from build123d import *

# Parameters (mm, degrees)
SKETCH_1_R                      = 1.440775231
EXTRUDE_1_DEPTH                 = 5
SKETCH_3_W                      = 35
SKETCH_3_H                      = 4
EXTRUDE_2_DEPTH                 = 50
FILLET_1_R                      = 10
FILLET_2_R                      = 5
CUT_EXTRUDE_2_DEPTH             = 63.339794674
CUT_EXTRUDE_2_DEPTH_BACK        = 63.339794674
CUT_EXTRUDE_3_REACH             = 64.34
SKETCH_5_R                      = 1.7
SKETCH_5_W                      = 10
SKETCH_5_H                      = 2.5
CUT_EXTRUDE_3_DIRECTION_2_DEPTH = 63.339794674
FILLET_3_R                      = 0.5
FILLET_4_R                      = 1


with BuildPart() as part:
    # 草图1 → 凸台-拉伸1 (new body)
    with BuildSketch(Plane.XY):
        with BuildLine():
            Line((-26, -2.5), (26, -2.5))
            ThreePointArc((26, -2.5), (28.5, 0), (26, 2.5))
            Line((26, 2.5), (20, 5))
            Line((20, 5), (-20, 5))
            Line((-20, 5), (-26, 2.5))
            ThreePointArc((-26, 2.5), (-28.5, 0), (-26, -2.5))
        make_face()
        with Locations((-26, 0)):
            Circle(SKETCH_1_R, mode=Mode.SUBTRACT)
        with Locations(Location((26, 0, 0), (0, 0, 180))):
            Circle(SKETCH_1_R, mode=Mode.SUBTRACT)
    extrude(amount=EXTRUDE_1_DEPTH)

    # 草图3 → 凸台-拉伸2 (add)
    with BuildSketch(Plane.XY.offset(5)):
        Rectangle(SKETCH_3_W, SKETCH_3_H)
    extrude(amount=EXTRUDE_2_DEPTH)

    # 圆角1
    # the kernel refuses this fillet: 10 mm, written as the material it adds along each edge
    with BuildSketch(Plane(origin=(17.5, -2, 5), x_dir=(0, -1.0, 2.1849189124477904e-12), z_dir=(-1, 0, 0))) as fillet_1_piece_1:
        with BuildLine():
            CenterArc((10, 3.122498999), FILLET_1_R, 180, 18.194872339)
            Line((0, 3.122498999), (-0.2, 3.122498999))
            Line((-0.2, 3.122498999), (-0.2, 0))
            Line((-0.2, 0), (0, -0.2))
            ThreePointArc((0, -0.2), (0.25, -0.2), (0.31, -0.06244998))
            Line((0.31, -0.06244998), (0.5, 0))
        make_face()
    extrude(amount=35)

    # 圆角2
    # the kernel refuses this fillet: 5 mm, written as the material it adds along each edge
    with BuildSketch(Plane(origin=(-17.5, 2, 5), x_dir=(0, 0, 1), z_dir=(1, 0, 0))) as fillet_2_piece_1:
        with BuildLine():
            CenterArc((4.582575695, -5), FILLET_2_R, 90, 66.421821522)
            Line((0, -3), (-0.091651514, -2.96))
            ThreePointArc((-0.091651514, -2.96), (-0.1, -1.5), (-0.1, 0))
            Line((-0.1, 0), (0, 0.1))
            Line((0, 0.1), (4.582575695, 0.1))
            Line((4.582575695, 0.1), (4.582575695, 0))
        make_face()
    extrude(amount=35)

    # 草图4 → 切除-拉伸2 (cut, two sides: drawn at the far end of the back side and taken through both)
    with BuildSketch(Plane.XZ.offset(2).offset(-CUT_EXTRUDE_2_DEPTH_BACK)):
        Polygon((-17.5, 51), (-13.5, 55), (-17.5, 55), align=None)
        Polygon((-13.5, 23), (-17.5, 27), (-17.5, 5), (-15.5, 5.511275368), (-10.5, 5.511275368), (-7.888776369, 8.122498999), (-7.888776369, 20.122498999), (-10.5, 23), align=None)
        Polygon((17.5, 5), (17.5, 27), (13.5, 23), (10.5, 23), (7.888776369, 20.122498999), (7.888776369, 8.122498999), (10.5, 5.511275368), (15.5, 5.511275368), align=None)
        Polygon((17.5, 51), (17.5, 55), (13.5, 55), align=None)
    extrude(amount=CUT_EXTRUDE_2_DEPTH + CUT_EXTRUDE_2_DEPTH_BACK, mode=Mode.SUBTRACT)

    # 草图5 → 切除-拉伸3 (cut, up to next)
    with BuildSketch(Plane.XZ.offset(2), mode=Mode.PRIVATE) as cut_extrude_3_sk1:
        with Locations(Location((-11.5, 26.128065597, 0), (0, 0, 180))):
            Circle(SKETCH_5_R)
    cut_extrude_3_tool1 = extrude(cut_extrude_3_sk1.sketch, amount=-CUT_EXTRUDE_3_REACH, mode=Mode.PRIVATE) & part.part
    # 草图5 → 切除-拉伸3 (cut, up to next)
    with BuildSketch(Plane.XZ.offset(2), mode=Mode.PRIVATE) as cut_extrude_3_sk2:
        with Locations(Location((11.5, 26.128065597, 0), (0, 0, 180))):
            Circle(SKETCH_5_R)
    cut_extrude_3_tool2 = extrude(cut_extrude_3_sk2.sketch, amount=-CUT_EXTRUDE_3_REACH, mode=Mode.PRIVATE) & part.part
    # 草图5 → 切除-拉伸3 (cut, up to next)
    with BuildSketch(Plane.XZ.offset(2), mode=Mode.PRIVATE) as cut_extrude_3_sk3:
        with Locations(Location((11.5, 51.128065597, 0), (0, 0, 180))):
            Circle(SKETCH_5_R)
    cut_extrude_3_tool3 = extrude(cut_extrude_3_sk3.sketch, amount=-CUT_EXTRUDE_3_REACH, mode=Mode.PRIVATE) & part.part
    # 草图5 → 切除-拉伸3 (cut, up to next)
    with BuildSketch(Plane.XZ.offset(2), mode=Mode.PRIVATE) as cut_extrude_3_sk4:
        with Locations(Location((-11.5, 51.128065597, 0), (0, 0, 180))):
            Circle(SKETCH_5_R)
    cut_extrude_3_tool4 = extrude(cut_extrude_3_sk4.sketch, amount=-CUT_EXTRUDE_3_REACH, mode=Mode.PRIVATE) & part.part
    # 草图5 → 切除-拉伸3 (cut, up to next)
    with BuildSketch(Plane.XZ.offset(2), mode=Mode.PRIVATE) as cut_extrude_3_sk5:
        with Locations((0, 13.122498999)):
            Rectangle(SKETCH_5_W, SKETCH_5_H)
    cut_extrude_3_tool5 = extrude(cut_extrude_3_sk5.sketch, amount=-CUT_EXTRUDE_3_REACH, mode=Mode.PRIVATE) & part.part
    add(cut_extrude_3_tool1.solids().sort_by_distance((-11.5, -2, 26.128066))[0], mode=Mode.SUBTRACT)
    add(cut_extrude_3_tool2.solids().sort_by_distance((11.5, -2, 26.128066))[0], mode=Mode.SUBTRACT)
    add(cut_extrude_3_tool3.solids().sort_by_distance((11.5, -2, 51.128066))[0], mode=Mode.SUBTRACT)
    add(cut_extrude_3_tool4.solids().sort_by_distance((-11.5, -2, 51.128066))[0], mode=Mode.SUBTRACT)
    add(cut_extrude_3_tool5.solids().sort_by_distance((0, -2, 13.122499))[0], mode=Mode.SUBTRACT)

    # 草图5 → 切除-拉伸3 direction 2 (cut)
    with BuildSketch(Plane.XZ.offset(2)):
        with Locations(Location((-11.5, 26.128065597, 0), (0, 0, 180))):
            Circle(SKETCH_5_R)
        with Locations(Location((11.5, 26.128065597, 0), (0, 0, 180))):
            Circle(SKETCH_5_R)
        with Locations(Location((11.5, 51.128065597, 0), (0, 0, 180))):
            Circle(SKETCH_5_R)
        with Locations(Location((-11.5, 51.128065597, 0), (0, 0, 180))):
            Circle(SKETCH_5_R)
        with Locations((0, 13.122498999)):
            Rectangle(SKETCH_5_W, SKETCH_5_H)
    extrude(amount=CUT_EXTRUDE_3_DIRECTION_2_DEPTH, mode=Mode.SUBTRACT)

    # 圆角3
    fillet_3_edges = [part.edges().sort_by_distance(p)[0] for p in [
        (5, 0, 11.872498999),
        (5, 0, 14.372498999),
        (-5, 0, 14.372498999),
        (-5, 0, 11.872498999),
    ]]
    fillet(fillet_3_edges, radius=FILLET_3_R)

    # 圆角4
    fillet_4_edges = [part.edges().sort_by_distance(p)[0] for p in [
        (17.5, 0, 51),
        (13.5, 0, 55),
        (17.5, 0, 27),
        (13.5, 0, 23),
        (10.5, 0, 23),
        (7.888776369, 0, 20.122498999),
        (7.888776369, 0.108965912, 8.122498999),
        (10.5, 0.875277907, 5.511275368),
        (15.5, 0.875277907, 5.511275368),
        (17.5, 1.25, 5),
        (-17.5, 1.25, 5),
        (-15.5, 0.875277907, 5.511275368),
        (-10.5, 0.875277907, 5.511275368),
        (-7.888776369, 0, 20.122498999),
        (-10.5, 0, 23),
        (-13.5, 0, 23),
        (-17.5, 0, 27),
        (-17.5, 0, 51),
        (-13.5, 0, 55),
    ]]
    fillet(fillet_4_edges, radius=FILLET_4_R)


solid = part.part
Geometry check sheet. Reference: the model listing, model coordinates, mm. A direction names the side the tool comes from. Round coordinates to 2 decimals unless told otherwise and drop trailing zeros. Order: outer loops, then holes, each group sorted by start corner. A loop starts at its lowest first (then second) coordinate and runs counter-clockwise, first axis right, second up. Notation, with made-up numbers: M 23.5,-26 L 54.5,-26 A3 ccw 54.5,-22 Z; hole C -4.5,42.5 d7. An arc over 180 degrees is marked long. Answer in a Markdown table with one row per item.
(1) Sectioned sample at A-A, the plane z = 32. Record the cut outline in (x, y).
Responses:
| item | result |
|---|---|
| outline | M -17.5,-2 L 17.5,-2 L 17.5,2 L -17.5,2 Z |
(2) Draft check along X on faces 1 (the face through (5, 0, 13)), 2 (the face through (28.5, -0.1, 2.5)), 3 (the face through (0, -2.5, 2)). Enter one of: released by +X, released by -X, zero draft, split by the parting line, or undercut.
Responses:
| item | result |
|---|---|
| face 1 | undercut |
| face 2 | released by +X |
| face 3 | zero draft |
(3) Tool access check on faces 4 (the face through (0, -2, 36)), 5 (the face through (0, 2, 37)). Record the directions out of +Z, -Z, +X, -X, +Y, -Y that give a thin tool (end or side, any length) a straight path to the whole face; none if there is none.
Responses:
| item | result |
|---|---|
| face 4 | +Z, +X, -X, -Y |
| face 5 | +Z, +X, -X, +Y |
